Part model, mm, in its own coordinate system. Coordinates: 2 decimals unless noted, no trailing zeros. Order: outer loops, then holes, each group sorted by start corner. A loop starts at its lowest first (then second) coordinate and runs counter-clockwise, first axis right, second up.
```python
from build123d import *

# Parameters (mm, degrees)
SKETCH1_R           = 9.5
SKETCH1_R_2         = 7.5
EXTRUDE_THIN1_DEPTH = 237


with BuildPart() as part:
    # Sketch1 → Extrude-Thin1 (new body)
    with BuildSketch(Plane(origin=(0, 0, 0), x_dir=(1, 0, 0), z_dir=(0, 1, 0))):
        Circle(SKETCH1_R)
        Circle(SKETCH1_R_2, mode=Mode.SUBTRACT)
    extrude(amount=EXTRUDE_THIN1_DEPTH)

    # Sketch6 → Cut-Revolve1 (revolve, cut)
    with BuildSketch(Plane(origin=(0, 0, 0), x_dir=(0, 0, -1), z_dir=(1, 0, 0))):
        Polygon((8.5, 8), (9.5, 8), (9.5, 10), align=None)
    revolve(axis=Axis((0, 8, -0.902354342), (0, 0, -1)), mode=Mode.SUBTRACT)

    # Sketch10 → Cut-Revolve3 (revolve, cut)
    with BuildSketch(Plane.XY):
        Polygon((9.5, 222), (9.5, 225), (8, 222), align=None)
    revolve(axis=Axis((18.348289419, 222, 0), (-1, 0, 0)), mode=Mode.SUBTRACT)


solid = part.part
```
(1) Probe line 1 (X direction, y = 126, z = 0); line 2 (X direction, y = 89.5, z = -2.75). List the from-to ranges inside material, lowest first.
(2) Slice it at A-A, the plane y = 121. Give the cut face in (x, z).
(3) Pull direction X, two halves, no side cores. Call faces 1 (the face through (4.38, 116.84, 8.43)), 2 (the face through (1, 237, -8)), 3 (the face through (-7.493, 116.841, -0.33)): +X half, -X half, draft (parallel to the pull), parting line (faces both ways), or undercut.
(4) Drop flat-ended pins along their axis: pin 1 (8 mm diameter, centred on y = 70.5, z = -6.5, fed in from +X); pin 2 (3 mm diameter, centred on x = -3, y = 153, fed in from +Z); pin 3 (3 mm diameter, centred on x = -5.5, z = 1.5, fed in from +Y). Give the stop position or say it passes through.
(5) Slice it at B-B, the plane z = 4.5. Give the cut face in (x, y), then the cut area to 3 significant figures.
Here are the results:
1. line 1: x = -9.5 to -7.5, 7.5 to 9.5
1. line 2: x = -9.09 to -6.98, 6.98 to 9.09
2. outline: circle Ø19 at (0, 0); hole circle Ø15 at (0, 0)
3. face 1: parting line
3. face 2: draft
3. face 3: undercut
4. pin 1: stops at x = 9.17
4. pin 2: stops at z = 9.38
4. pin 3: passes through
5. outline: (-8.37, 0) - (-6, 0) - (-6, 237) - (-8.37, 237) - close; (6, 0) - (8.37, 0) - (8.37, 237) - (6, 237) - close
5. area: 1,120 mm2
